Check sheet for the modelled part. Datum: model origin and axes. Units: mm. Face numbers are marked on the shaded views. Round coordinates to 2 decimals unless told otherwise and drop trailing zeros. Order: outer loops, then holes, each group sorted by start corner. A loop starts at its lowest first (then second) coordinate and runs counter-clockwise, first axis right, second up.
Q1. Cross-section at A-A on y = 87. Record the cut outline in (x, z), then the cut area to 3 significant figures.
Q2. Depth check by flat-ended pin: P1, Ø1, axis at x = 19, y = 93, coming from the +Z side; P2, Ø12, axis at y = 41, z = 12.5, coming from the -X side; P3, Ø1.5, axis at x = -5, y = 41.5, coming from the -Z side. Enter the tip coordinate at first touch or a pass-through.
Q3. Scan lines: probe 1 along Z at (x, y) = (-1.5, 18); probe 2 along Y at (x, z) = (27, 7); probe 3 along X at (y, z) = (120, -14). Record each from-to range of solid material in increasing order.
Q4. Mould release check, pull along X, two halves, no side actions. Record for the marked faces 1 and 2: +X half, -X half, draft (parallel to the pull), parting line (faces both ways), or undercut.
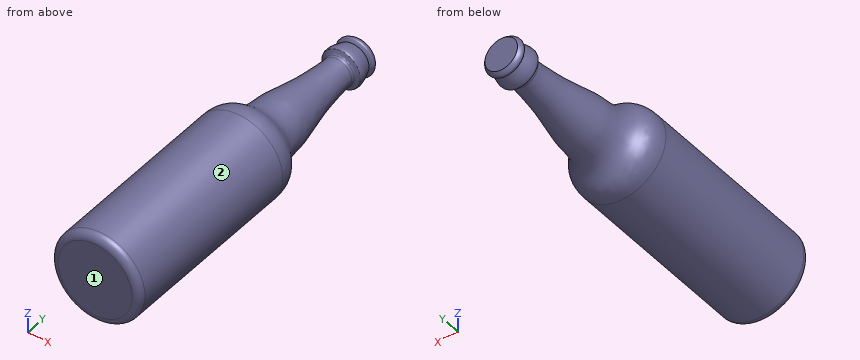
Autodesk Fusion 360 part; units mm, degrees
sketch "Sketch1" plane through (0, 0, 0) normal (0, 0, 1) x (1, 0, 0) in component "Bottle"
  line L0 (0, 0) -> (0, 240)
  line L1 (0, 0) -> (30, 0)
  line L2 (30, 0) -> (30, 130)
  spline S0 degree 5 poles (30, 130) (29.998, 130.5867) (29.9763, 131.7424) (29.891, 133.4228) (29.6561, 135.5533) (29.0844, 138.0165) (28.1655, 140.2736) (26.8747, 142.3415) (25.2854, 144.28) (23.5656, 146.1888) (21.9148, 148.1805) (20.5169, 150.3601) (19.4863, 152.8016) (18.8176, 155.5265) (18.4238, 158.5188) (18.171, 161.7388) (17.9157, 165.1381) (17.5383, 168.6723) (16.9848, 172.3181) (16.2605, 176.0711) (15.4096, 179.938) (14.4998, 183.9314) (13.6047, 188.0637) (12.7875, 192.3401) (12.0839, 196.7543) (11.4848, 201.279) (10.9562, 205.858) (10.4853, 210.3683) (10.0776, 214.649) (9.8642, 218.3732) (9.9543, 221.2857) (10.8878, 222.5808) (12.5552, 222.4718) (13.3816, 223.3082) (13.5145, 224.987) (13.1496, 227.29) (12.5016, 229.5972) (11.8316, 231.5704) (11.3023, 232.9949) (11.0171, 233.7344) knots 0 0 0 0 0 0 0.028571 0.057143 0.085714 0.114286 0.142857 0.171429 0.2 0.228571 0.257143 0.285714 0.314286 0.342857 0.371429 0.4 0.428571 0.457143 0.485714 0.514286 0.542857 0.571429 0.6 0.628571 0.657143 0.685714 0.714286 0.742857 0.771429 0.8 0.828571 0.857143 0.885714 0.914286 0.942857 0.971429 1 1 1 1 1 1
  line L3 (30.0435, 117.5044) -> (29.9565, 142.4956)
  line L4 (8.2601, 215.0919) -> (12.1986, 227.1701)
  line L5 (9.449, 218.6711) -> (16.5255, 227.5827)
  spline S1 degree 5 poles (11.0171, 233.7344) (11.4206, 233.9324) (12.1146, 234.3372) (12.817, 234.9704) (13.1658, 235.858) (12.9204, 237.0026) (12.3468, 237.9168) (11.742, 238.5879) (11.2604, 239.0266) (11, 239.2438) knots 0 0 0 0 0 0 0.2 0.4 0.6 0.8 1 1 1 1 1 1
  line L6 (11.4748, 238.8477) -> (10.5252, 239.6399)
  line L7 (10.3402, 233.4022) -> (11.6939, 234.0666)
  line L8 (11, 239.2438) -> (0, 239.2438)
  point P0 (27.4621, 141.314)
  point P1 (20.6353, 150.3726)
  point P2 (17.8039, 166.0148)
  point P3 (12.7238, 192.9048)
  point P4 (10.2294, 221.131)
  point P5 (12.9872, 223.1269)
  dimension "d1" = 240
  dimension "d2" = 30
  dimension "d3" = 130
  dimension "d7" = 11
revolve "Revolve1" add sketch "Sketch1" angle 360 about axis through (0, 0, 0) along (0, 1, 0) contours L0 L1 L2 S0 S1 L8 in component "Bottle"
fillet "Fillet1" radius 5 1 edges at (-27.9698, 0, -10.8485) in component "Bottle"
shell "Shell1" thickness 2.5 removed faces 1 at (2.9076, 239.2438, 1.5312) in component "Bottle"
component "Bottle" placed x (1, 0, 0) y (0, 1, 0) z (0, 0, 1) at (0, 0, 0)
Results found:
1. outline: circle Ø60 at (0, 0)
1. area: 2,830 mm2
2. P1: stops at z = 23.62
2. P2: stops at x = -29.29
2. P3: stops at z = -29.7
3. probe 1: z = -29.96 to 29.96
3. probe 2: y = 0.92 to 140.57
3. probe 3: x = -26.53 to 26.53
4. face 1: draft
4. face 2: parting line
